Autodesk Inventor part; units mm, degrees
ref_plane "XZ Plane" through (0, 0, 0) normal (0, 1, 0) x (-1, 0, 0)
ref_plane "XY Plane" through (0, 0, 0) normal (0, 0, 1) x (1, 0, 0)
ref_plane "Work Plane1" through (78.575, 0, 0) normal (1, 0, 0) x (0, 1, 0)
sketch "Sketch2" plane through (78.575, 0, 0) normal (1, 0, 0) x (0, 1, 0)
  line L0 (-170.29, 0) -> (141.6673, 38.3035)
  line L1 (141.6673, 38.3035) -> (140.4486, 48.229)
  line L2 (-171.5087, 9.9255) -> (140.4486, 48.229)
  line L3 (-170.29, 0) -> (-171.5087, 9.9255)
  line L4 (-304.8, 0) -> (304.8, 0)
  line L5 (-304.8, 0) -> (-304.8, -25.4)
  line L6 (304.8, -25.4) -> (-304.8, -25.4)
  line L7 (304.8, 0) -> (304.8, -25.4)
  line L8 (141.6673, 0) -> (146.6673, 0)
  line L9 (146.6673, 0) -> (146.6673, 53.4221)
  line L10 (146.6673, 53.4221) -> (141.6673, 53.4221)
  line L11 (141.6673, 53.4221) -> (141.6673, 0)
  line L12 (141.6673, 53.4221) -> (121.6673, 53.4221)
  line L13 (121.6673, 53.4221) -> (121.6673, 38.3035)
  line L14 (121.6673, 38.3035) -> (141.6673, 38.3035)
  line L15 (141.6673, 38.3035) -> (141.6673, 53.4221)
  line L16 (141.6673, 38.3035) -> (140.4486, 48.229)
  line L17 (121.6673, 45.8628) -> (140.4486, 48.229)
  line L18 (146.6673, 0) -> (96.6673, 0)
  line L19 (96.6673, 0) -> (96.6673, 5)
  line L20 (96.6673, 5) -> (146.6673, 5)
  line L21 (146.6673, 5) -> (146.6673, 0)
  line L22 (141.6673, 53.4221) -> (121.6673, 50.9023)
  line L23 (101.6673, 0) -> (141.6673, 0)
  line L24 (141.6673, 0) -> (141.6673, 0.65)
  line L25 (141.6673, 0.65) -> (101.6673, 0.65)
  line L26 (101.6673, 0.65) -> (101.6673, 0)
  point P0 (0, 0)
  point P1 (141.6673, 5)
  point P2 (121.6673, 45.9229)
  point P3 (141.6673, 0.65)
  dimension "d2" = 5
  dimension "d3" = 20
  dimension "d4" = 50
  dimension "d5" = 5
  dimension "d6" = 5
  dimension "d7" = 40
  dimension "d8" = 5
  dimension "d9" = 0.65
extrude "Extrusion1" add sketch "Sketch2" along normal mid plane 25 contours L1 L2 L13 L22 L11 | L11 L10 L9 L20 | L19 L20 L11 L25 L26 L4 | L20 L9 L4 L11 | L26 L25 L11 L4
extrude "Extrusion2" cut sketch "Sketch2" along normal mid plane 13.2 contours L26 L25 L11 L4
fillet "Fillet1" radius 31.25 1 edges at (78.575, 141.6673, 5)
properties part number "coverHolder"
Input: part model. Units: mm. Frame: model coordinates. A direction names the side the tool comes from. Round coordinates to 2 decimals unless told otherwise and drop trailing zeros. Order: outer loops, then holes, each group sorted by start corner. A loop starts at its lowest first (then second) coordinate and runs counter-clockwise, first axis right, second up. Notation, with made-up numbers: (74.25, -29.5) - (124.25, -29.5) arc R18 cw to (124.25, -22.5) - close; hole circle Ø3 at (54.25, 42). An arc over 180 degrees is marked (long way). Use a Markdown table: item, result.
1. Section D-D on x = 77.5. Return the cut outline in (y, z).
Evaluation:
| item | result |
|---|---|
| outline | (96.67, 0) - (101.67, 0) - (101.67, 0.65) - (141.67, 0.65) - (141.67, 0) - (146.67, 0) - (146.67, 53.42) - (141.67, 53.42) - (121.67, 50.9) - (121.67, 45.92) - (140.45, 48.23) - (141.67, 38.3) - (141.67, 36.25) arc R31.25 cw to (110.42, 5) - (96.67, 5) - close |
2. Section A-A on y = 109.5. Return the cut outline in (x, z) (3 decimals), then the cut area to 3 significant figures.
Evaluation:
| item | result |
|---|---|
| outline | (66.075, 0) - (71.975, 0) - (71.975, 0.65) - (85.175, 0.65) - (85.175, 0) - (91.075, 0) - (91.075, 5) - (66.075, 5) - close |
| area | 116 mm^2 |
3. First-contact query: pin 1 (12 mm diameter, centred on x = 81, y = 134.5, fed in from +Z); pin 2 (10 mm diameter, centred on x = 76, y = 104.5, fed in from -Z); pin 3 (2.5 mm diameter, centred on x = 83, z = 37.5, fed in from -Y); pin 4 (6.5 mm diameter, centred on x = 77.5, y = 116.5, fed in from -Z). Flat tips, straight axial feed; report the tip coordinate or a pass-through.
Evaluation:
| item | result |
|---|---|
| pin 1 | z = 53.28 |
| pin 2 | z = 0 |
| pin 3 | y = 141.61 |
| pin 4 | z = 0.65 |
4. Mould query, pull axis Z, two halves, no side actions, for faces 1 (the face through (78, 141.667, 37)), 2 (the face through (70, 121, 0)), 3 (the face through (78.4, 131.81, 52.18)), 4 (the face through (78, 121.667, 48)). Classes: +Z half, -Z half, draft (parallel to the pull), parting line (faces both ways), or undercut.
Evaluation:
| item | result |
|---|---|
| face 1 | undercut |
| face 2 | -Z half |
| face 3 | +Z half |
| face 4 | draft |
5. Section B-B on x = 71. Return the cut outline in (y, z).
Evaluation:
| item | result |
|---|---|
| outline | (96.67, 0) - (146.67, 0) - (146.67, 53.42) - (141.67, 53.42) - (121.67, 50.9) - (121.67, 45.92) - (140.45, 48.23) - (141.67, 38.3) - (141.67, 36.25) arc R31.25 cw to (110.42, 5) - (96.67, 5) - close |
6. Access query for faces 5 (the face through (78.4, 130.93, 47.06)), 6 (the face through (78.75, 132.27, 13.91)), 7 (the face through (78, 103, 5)), 8 (the face through (78, 122, 0.65)), 9 (the face through (78, 96.667, 2)). Directions: +Z, -Z, +X, -X, +Y, -Y. A direction counts if a zero-diameter tool reaches every point of the face in a straight line with its end or side. Return the directions, or none.
Evaluation:
| item | result |
|---|---|
| face 5 | +X, -X |
| face 6 | +X, -X, -Y |
| face 7 | +Z, +X, -X, -Y |
| face 8 | -Z |
| face 9 | +Z, -Z, +X, -X, -Y |
7. Section C-C on y = 134.5. Return the cut outline in (x, z) (3 decimals), then the cut area to 3 significant figures.
Evaluation:
| item | result |
|---|---|
| outline | (66.075, 0) - (71.975, 0) - (71.975, 0.65) - (85.175, 0.65) - (85.175, 0) - (91.075, 0) - (91.075, 16.336) - (66.075, 16.336) - close; (66.075, 47.499) - (91.075, 47.499) - (91.075, 52.519) - (66.075, 52.519) - close |
| area | 525 mm^2 |
8. Material intervals for probe 1 along Y at (x, z) = (73.25, 38); probe 2 along Z at (x, y) = (69, 102); probe 3 along Z at (x, y) = (88.25, 128), sorted ascending.
Evaluation:
| item | result |
|---|---|
| probe 1 | 141.67 to 146.67 |
| probe 2 | 0 to 5 |
| probe 3 | 0 to 10.42, 46.7 to 51.7 |
